from build123d import *

# Parameters (mm, degrees)
F2_W     = 20.069398
F2_H     = 8.830535
F3_DEPTH = 6350


with BuildPart() as f1:
    # F0 (on Front) → F1 (revolve)
    with BuildSketch(Plane.XZ):
        Polygon((0, -13.245802), (0, 0), (28.36475, 0), (28.36475, 3.612492), (34.251776, 3.612492), (34.251776, 8.429147), (0, 8.429147), (0, 16.456908), (-8.295352, 16.456908), (-8.295352, 8.429147), (-60.208194, 8.429147), (-60.208194, 11.105067), (-68.771139, 11.105067), (-68.771139, 6.288412), (-45.758229, 6.288412), (-45.758229, 0), (-8.295352, 0), (-8.295352, -13.245802), align=None)
    revolve(axis=Axis((-4.147676, 0, -13.245802), (-1, 0, 0)))

    # F2 (on Front) → F3 (cut, symmetric)
    with BuildSketch(Plane.XZ):
        with Locations((-62.482726, -13.379599)):
            Rectangle(F2_W, F2_H)
    extrude(amount=F3_DEPTH, both=True, mode=Mode.SUBTRACT)


solid = f1.part
Geometry check sheet. Reference: the model listing, model coordinates, mm. A direction names the side the tool comes from. Give positions to 0.01 mm unless a question says otherwise; leave off trailing zeros. Order: outer loops, then holes, each group sorted by start corner. A loop starts at its lowest first (then second) coordinate and runs counter-clockwise, first axis right, second up.
1) Gauge pin test, flat ends, axial feed: pin 1 (8 mm diameter, centred on y = -3, z = -21.5, fed in from -X); pin 2 (4 mm diameter, centred on x = -24, y = 16.5, fed in from +Z); pin 3 (2.5 mm diameter, centred on x = -58, y = -20.5, fed in from -Z). Record the tip position at first contact, or that the pin passes through.
Results are:
pin 1: stops at x = -8.3
pin 2: stops at z = 2.86
pin 3: stops at z = -23.21
2) Material ranges on probe 1 along Z at (x, y) = (-56, 0); probe 2 along X at (y, z) = (-1.5, 10.5); probe 3 along X at (y, z) = (-5.5, -27), recorded low to high.
Results are:
probe 1: z = -34.92 to -32.78, 6.29 to 8.43
probe 2: x = -68.77 to -60.21, -8.3 to 0
probe 3: x = -45.76 to 28.36
3) Tool access check on faces 1 (the flat face through (-60.208, -2, 9)), 2 (the flat face through (-8.295, 0, -13)), 3 (the cylindrical face through (-64.55, 0.471, -37.592)), 4 (the flat face through (-52.448, 20, -13)), 5 (the flat face through (28.365, -9, -3)). Record the directions out of +Z, -Z, +X, -X, +Y, -Y that give a thin tool (end or side, any length) a straight path to the whole face; none if there is none.
Results are:
face 1: +Z
face 2: -X
face 3: -Z, -X
face 4: -X, +Y, -Y
face 5: +X
4) Draft check along Y on faces 6 (the flat face through (34.252, -11, 0)), 7 (the cylindrical face through (14.38, -5.07, -1.01)), 8 (the cylindrical face through (16.89, 14.65, -29.22)). Enter one of: released by +Y, released by -Y, zero draft, split by the parting line, or undercut.
Results are:
face 6: zero draft
face 7: undercut
face 8: split by the parting line
5) Cross-section at D-D (x = -3). Record the boundary of the cut face in (y, z), then the cut area to 3 significant figures.
Results are:
outline: circle Ø59.41 at (0, -13.25)
area: 2,770 mm2
6) Cross-section at C-C (x = -31.5). Record the boundary of the cut face in (y, z).
Results are:
outline: circle Ø43.35 at (0, -13.25); hole circle Ø26.49 at (0, -13.25)
